Source: CAD feature listing. Evaluate the final solid. Frame: model axes, mm. A direction names the side the tool comes from. Coordinates: 2 decimals unless noted, no trailing zeros. Order: outer loops, then holes, each group sorted by start corner. A loop starts at its lowest first (then second) coordinate and runs counter-clockwise, first axis right, second up.
Autodesk Inventor part; units mm, degrees
ref_plane "Work Plane1" through (32.4111, 0, 0) normal (0, 0, -1) x (-1, 0, 0)
ref_plane "YZ Plane" through (0, 0, 0) normal (1, 0, 0) x (0, 1, 0)
ref_plane "XZ Plane" through (0, 0, 0) normal (0, 1, 0) x (-1, 0, 0)
sketch "Boceto1" plane through (0, 0, 0) normal (0, 0, 1) x (1, 0, 0)
  line L0 (-2.3053, 0) -> (12.0509, 0)
  line L1 (4.0411, 7.5) -> (2.8595, 10.0339)
  line L2 (4.0411, 7.5) -> (10, 7.5) construction
  line L3 (10, 7.5) -> (10, 0) construction
  arc A0 (2.8595, 10.0339) -> (0, 9.4) centre (1.5, 9.4) ccw
  line L4 (4.0411, 7.5) -> (4.0411, 0)
  line L5 (0, -2.2363) -> (0, 13.4177)
  point P0 (0, 0)
  dimension "d2" = 15
  dimension "d4" = 21.8
  dimension "d5" = 1.5
  dimension "d15" = 10
  dimension "d16" = 25
revolve "Anilla" add sketch "Boceto1" angle 360 about axis through (-10, 0, 0) along (1, 0, 0)
sketch "Boceto2" plane through (0, 0, 0) normal (-1, 0, 0) x (0, 0, 1)
  circle A0 centre (0, 0) radius 4.9
  line L0 (-7.5, -4.3301) -> (-7.5, 4.3301)
  line L1 (-7.5, 4.3301) -> (0, 8.6603)
  line L2 (0, 8.6603) -> (7.5, 4.3301)
  line L3 (7.5, 4.3301) -> (7.5, -4.3301)
  line L4 (7.5, -4.3301) -> (0, -8.6603)
  line L5 (0, -8.6603) -> (-7.5, -4.3301)
  circle A1 centre (0, 0) radius 9.4
  dimension "d6" = 17.3205
extrude "Cuerpo" add sketch "Boceto2" against normal blind 10 contours A0 | L0 L1 L2 L3 L4 L5
sketch "Boceto3" plane through (0, 0, 0) normal (0, 0, 1) x (1, 0, 0)
  line L0 (3.5, 8.6603) -> (10, 8.6603)
  line L1 (10, 4.3301) -> (10, 8.6603)
  line L2 (0, -9.4) -> (0, 9.4)
  line L3 (-2, 0) -> (12, 0)
  line L4 (9.3301, 8.6603) -> (10, 7.5)
  dimension "d10" = 30
  dimension "d11" = 15
revolve "Chaflán1" cut sketch "Boceto3" angle 360 about axis through (-10, 0, 0) along (1, 0, 0)
sketch "Boceto4" plane through (0, 0, 0) normal (-1, 0, 0) x (0, 0, 1)
  circle A0 centre (0, 0) radius 9.4
hole "Rosca" at (0, 0, 0) direction (1, 0, 0) diameter 8.376 end through all
chamfer "Chaflán2" distance 0.8119 angle 30 1 edges at (0, 0, -4.188) measured on face at (0, 7.5614, -0.9181)
ref_plane "Work Plane1" through (32.4111, 0, 0) normal (0, 0, -1) x (-1, 0, 0)
chamfer "Chaflán3" distance 0.8119 angle 45 1 edges at (10, 0, -4.188)
equation "\"d2\" = SW"
equation "\"d4\" = LADI"
equation "\"d5\" = PHH"
equation "\"d15\" = KOH"
equation "\"d16\" = KEWI"
equation "\"d6\" = 1.1547 * SW"
equation "\"d7\" = KOH"
equation "\"d10\" = ANG1"
equation "\"d11\" = SW0"
equation "\"d12\" = -0.5 * GD1 + 0.5 * NND"
equation "\"d46\" = -0.5 * GD1 + 0.5 * NND"
equation "\"d51\" = -0.5 * GD1 + 0.5 * NND"
equation "\"ANG1\" = 30deg"
equation "\"KEWI\" = 25deg"
equation "\"LADI\" = 21.8"
equation "\"SW\" = 15"
equation "\"PHH\" = 1.5"
equation "\"KOH\" = NND"
equation "\"SW0\" = 15"
equation "\"d1\" = LADI"
equation "\"d3\" = PHH"
equation "\"GUL\" = 0.541266 * PTC"
equation "\"RR\" = PHH"
equation "\"TOA\" = 30deg"
equation "\"PTC\" = 1.5"
equation "\"GAL\" = 0.541266 * PTC"
equation "\"E0\" = 1.155 * SW"
properties part number "ISO 4161 - M10" material "Acero inoxidable"
1. Section query B-B, the plane x = 1.25. Output: boundary loops of the cut face in (y, z).
2. Section query A-A, the plane x = 6. Output: boundary loops of the cut face in (y, z), plus the area to 3 significant figures.
3. Access query for faces 4 (the flat face through (6.705, 6.526, 3.698)), 5 (the conical face through (9.84, 7.78, 0.02)), 6 (the flat face through (6.705, -6.526, -3.698)). Directions: +Z, -Z, +X, -X, +Y, -Y. A direction counts if a zero-diameter tool reaches every point of the face in a straight line with its end or side. Return the directions, or none.
4. Contact query for flat-ended pins moving along their axis: P1, Ø6, axis at y = -7.5, z = 7, coming from the -X side; P2, Ø1.5, axis at x = 6.5, y = 3, coming from the +Z side; P3, Ø2, axis at y = -1.5, z = 3, coming from the +X side; P4, Ø3, axis at y = 1.5, z = 3, coming from the -X side. Output: stop coordinate, or through.
5. Material intervals for line 1 along Z through (x, y) = (5.5, 0); line 2 along Y through (x, z) = (1.25, 0.25); line 3 along Z through (x, y) = (9.25, -1.5), sorted ascending.
6. Draft query along Z for faces 1 (the flat face through (6.705, -6.465, 3.803)), 2 (the flat face through (6.705, 6.465, -3.803)), 3 (the cylindrical face through (4.889, -2.83, -3.087)). Return one class per face: +Z half, -Z half, draft (parallel to the pull), parting line (faces both ways), or undercut.
Answer key:
1. outline: circle Ø21.76 at (0, 0); hole circle Ø8.38 at (0, 0)
2. outline: (-8.66, 0) - (-4.33, -7.5) - (4.33, -7.5) - (8.66, 0) - (4.33, 7.5) - (-4.33, 7.5) - close; hole circle Ø8.38 at (0, 0)
2. area: 140 mm2
3. face 4: +Z, +X, +Y
3. face 5: +X, +Y
3. face 6: -Z, +X, -Y
4. P1: stops at x = 0
4. P2: stops at z = 7.5
4. P3: stops at x = 9.35
4. P4: stops at x = 0.08
5. line 1: z = -7.5 to -4.19, 4.19 to 7.5
5. line 2: y = -10.88 to -4.18, 4.18 to 10.88
5. line 3: z = -7.5 to -3.98, 3.98 to 7.5
6. face 1: +Z half
6. face 2: -Z half
6. face 3: undercut
